Part model, mm, in its own coordinate system. A direction names the side the tool comes from. Round coordinates to 2 decimals unless told otherwise and drop trailing zeros. Loops run counter-clockwise (first coordinate to the right, second up) from the corner with the lowest first, then second, coordinate; pieces in that order, holes last. Notation, with made-up numbers: M 17,-30.75 L 28,-30.75 A23 cw 28,-17.75 Z; hole C 27,70.25 d7. An arc over 180 degrees is marked long. Answer as CSV lines item,"result". Start each with the question number.
Item 1: Band-saw the part on C-C (x = 8). Give the cut face in (y, z), and give its area (3 significant figures).
Item 2: Drop flat-ended pins along their axis: pin 1 Ø2 at (y, z) = (-6.5, 2) entering from +X; pin 2 Ø0.6 at (x, z) = (15.5, 3) entering from +Y; pin 3 Ø1.5 at (x, z) = (7, 3.5) entering from -Y; pin 4 Ø2 at (y, z) = (0, 3) entering from -X. Give the stop position or say it passes through.
Item 3: Band-saw the part on A-A (y = -1.5). Give the cut face in (x, z), and give its area (3 significant figures).
Item 4: Which spindle directions (+Z, -Z, +X, -X, +Y, -Y) get a long thin tool onto all of the face, cutting with end or side? Do faces 1 (the flat face through (18.3, 0, 1.55)), 2 (the flat face through (13.1, 0, 3)), 3 (the flat face through (16, -3.95, 3)), 4 (the flat face through (16, 3.95, 3)), 5 (the flat face through (18.85, 0, 3)). Say none if no direction does.
Item 5: Band-saw the part on B-B (z = 2.8). Give the cut face in (x, y).
Item 6: Wall check: line 1 (Z direction, x = -0.5, y = -8); line 2 (X direction, y = -1.5, z = 3.45); line 3 (Y direction, x = 13.5, z = 2). Give the ranges that are in metal, low to high.
```python
from build123d import *

# Parameters (mm, degrees)
F0_W     = 35.7
F0_H     = 18
F1_DEPTH = 1.55
F2_W     = 5.75
F2_H     = 7.9
F3_DEPTH = 2.75
F4_R     = 0.75


with BuildPart() as f1:
    # F0 (on Top) → F1 (new body)
    with BuildSketch(Plane.XY):
        Rectangle(F0_W, F0_H)
    extrude(amount=F1_DEPTH)

    # F2 (on face) → F3 (join)
    with BuildSketch(Plane.XY.offset(1.55)):
        with Locations((15.975, 0)):
            Rectangle(F2_W, F2_H)
    extrude(amount=F3_DEPTH)

    # F4
    f4_edges = [f1.edges().sort_by_distance(p)[0] for p in [
        (15.975, 3.95, 4.3),
        (15.975, -3.95, 4.3),
        (18.35, 3.95, 1.55),
        (18.35, -3.95, 1.55),
    ]]
    fillet(f4_edges, radius=F4_R)


solid = f1.part
```
Answer block:
1,outline,"M -9,0 L 9,0 L 9,1.55 L -9,1.55 Z"
1,area,"27.9 mm^2"
2,pin 1,"stops at x = 17.85"
2,pin 2,"stops at y = 3.95"
2,pin 3,"passes through"
2,pin 4,"stops at x = 13.1"
3,outline,"M -17.85,0 L 17.85,0 L 17.85,1.55 L 18.85,1.55 L 18.85,4.3 L 13.1,4.3 L 13.1,1.55 L -17.85,1.55 Z"
3,area,"71.1 mm^2"
4,face 1,"-Z, +X, +Y, -Y"
4,face 2,"+Z, -X, +Y, -Y"
4,face 3,"+Z, +X, -X, -Y"
4,face 4,"+Z, +X, -X, +Y"
4,face 5,"+Z, -Z, +X, +Y, -Y"
5,outline,"M 13.1,-3.95 L 18.85,-3.95 L 18.85,3.95 L 13.1,3.95 Z"
6,line 1,"z = 0 to 1.55"
6,line 2,"x = 13.1 to 18.85"
6,line 3,"y = -3.95 to 3.95"
